Part model, mm, in its own coordinate system. Face numbers are marked on the shaded views. A direction names the side the tool comes from. Give positions to 0.01 mm unless a question says otherwise; leave off trailing zeros. Write each loop counter-clockwise with the first axis right and the second up, starting at its lowest first coordinate (ties: lowest second). Pieces come first, ordered by that corner, then holes.
from build123d import *

# Parameters (mm, degrees)
SKETCH1_R           = 12
BOSS_EXTRUDE1_DEPTH = 24
SKETCH2_R           = 5
CUT_EXTRUDE1_DEPTH  = 12
SKETCH3_R           = 6
BOSS_EXTRUDE2_DEPTH = 20


with BuildPart() as part:
    # Sketch1 → Boss-Extrude1 (new body)
    with BuildSketch(Plane.XY):
        Circle(SKETCH1_R)
    extrude(amount=BOSS_EXTRUDE1_DEPTH)

    # Sketch2 → Cut-Extrude1 (cut)
    with BuildSketch(Plane.XY.offset(24)):
        Circle(SKETCH2_R)
    extrude(amount=-CUT_EXTRUDE1_DEPTH, mode=Mode.SUBTRACT)

    # Sketch3 → Boss-Extrude2 (add)
    with BuildSketch(Plane(origin=(0, 0, 0), x_dir=(-1, 0, 0), z_dir=(0, 0, -1))):
        Circle(SKETCH3_R)
    extrude(amount=BOSS_EXTRUDE2_DEPTH)


solid = part.part
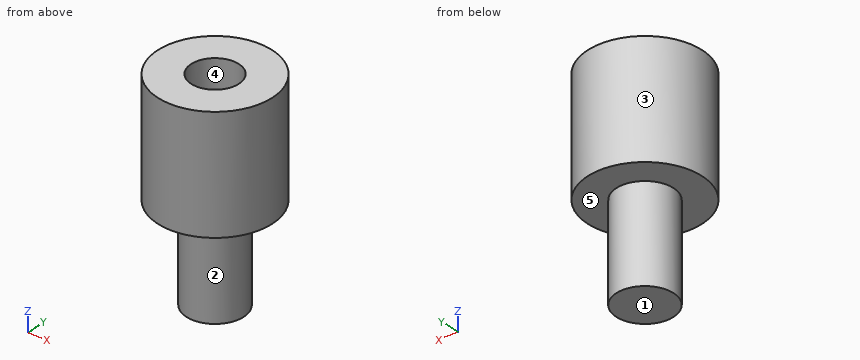
1) Saw through at C-C (z = -9.5). Write the cut outline in (x, y), and give its area (3 significant figures).
Check result:
outline: circle Ø12 at (0, 0)
area: 113 mm2
2) Flat gauge pins, fed straight in: P1, Ø4, axis at x = -3.5, y = -6.5, coming from the -Z side; P2, Ø6, axis at x = 0, y = 0, coming from the +Z side; P3, Ø1, axis at y = -1, z = -4, coming from the +X side; P4, Ø1.5, axis at y = -8.5, z = -3.5, coming from the -X side. Where does each tip first touch, or does it go through?
Check result:
P1: stops at z = -20
P2: stops at z = 12
P3: stops at x = 5.98
P4: passes through
3) Saw through at A-A (y = 0). Write the cut outline in (x, z).
Check result:
outline: (-12, 0) - (-6, 0) - (-6, -20) - (6, -20) - (6, 0) - (12, 0) - (12, 24) - (5, 24) - (5, 12) - (-5, 12) - (-5, 24) - (-12, 24) - close
4) Saw through at D-D (y = -8.5). Write the cut outline in (x, z).
Check result:
outline: (-8.47, 0) - (8.47, 0) - (8.47, 24) - (-8.47, 24) - close
5) 3-axis set-ups, long thin cutter, end or side, ignore diameter. For the marked faces 1 and 2: which of +Z, -Z, +X, -X, +Y, -Y reach the whole face in a straight line?
Check result:
face 1: -Z, +X, -X, +Y, -Y
face 2: -Z
6) Mould opens along Y. For the marked faces 3, 4 and 5 say: +Y half, -Y half, draft (parallel to the pull), parting line (faces both ways), or undercut.
Check result:
face 3: parting line
face 4: undercut
face 5: draft
7) Drill centre lines: L1, parallel to Y at x = 0, z = 14.75; L2, parallel to Z at x = 5, y = 10.5; L3, parallel to Z at x = 0, y = 3.5. Where is each one in solid material? Low to high.
Check result:
L1: y = -12 to -5, 5 to 12
L2: z = 0 to 24
L3: z = -20 to 12
